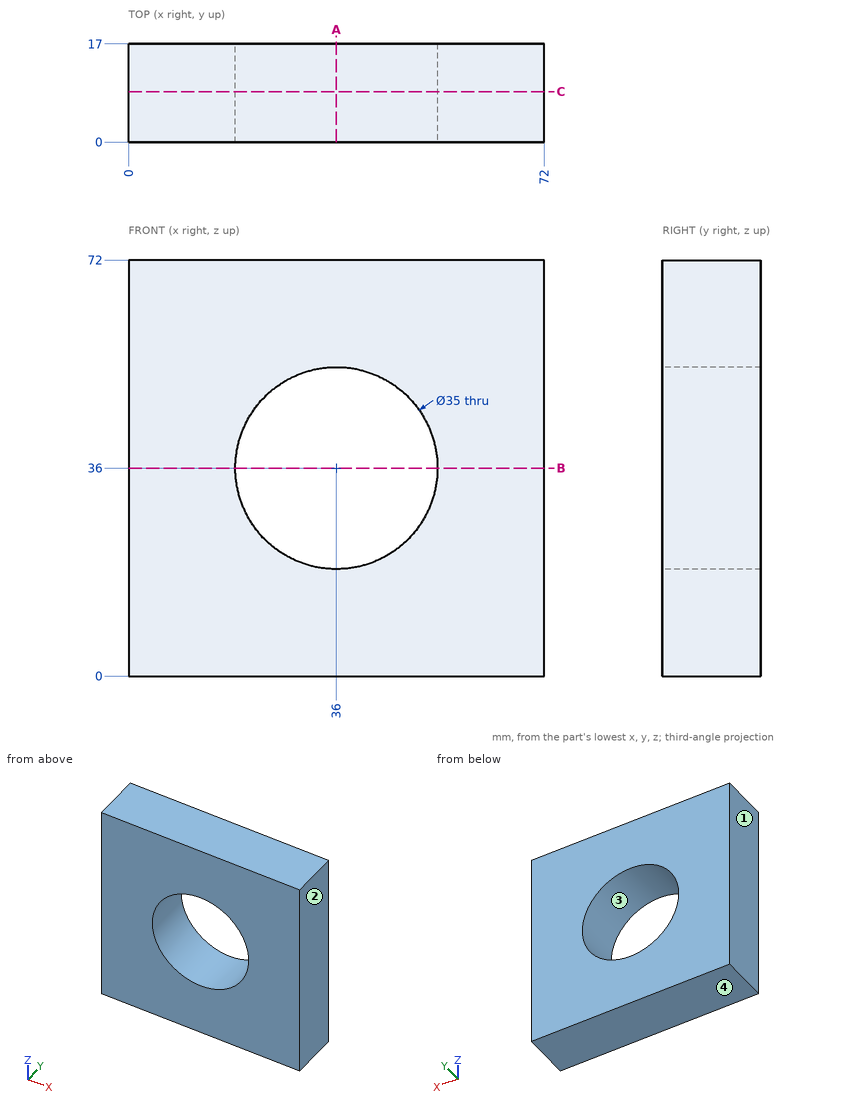
Geometry: see drawing. Coordinates: mm, zero at the bounding-box minimum. Give positions to 0.01 mm unless a question says otherwise; leave off trailing zeros. Loops run counter-clockwise (first coordinate to the right, second up) from the corner with the lowest first, then second, coordinate; pieces in that order, holes last. Notation, with made-up numbers: (31.25, 8.25) -> (85.25, 8.25) arc R34 ccw to (85.25, 46.25) -> close; hole circle Ø6 at (27, 64). An arc over 180 degrees is marked (long way). Put each result on its own line as item: value.
1. Pin query (flat end, axial travel): P1, Ø5, axis at x = 46.5, y = 5.5, coming from the -Z side. Return the tip coordinate at first contact, or that it passes through.
Taken from the geometry:
P1: stops at z = 0
2. Pull-direction query (X, two-part tool) for the marked faces 1, 2, 3 and 4; classes: released by +X, released by -X, zero draft, split by the parting line, or undercut.
Taken from the geometry:
face 1: released by -X
face 2: released by +X
face 3: undercut
face 4: zero draft
3. Ray query, line 1 along Z through (x, y) = (36, 7.75); line 2 along X through (y, z) = (12.5, 28); line 3 along X through (y, z) = (7.5, 23.5). Return the intervals inside material, ascending. Write a range as [from, to].
Taken from the geometry:
line 1: z = [0, 18.5], [53.5, 72]
line 2: x = [0, 20.44], [51.56, 72]
line 3: x = [0, 23.75], [48.25, 72]
4. Cut plane B-B (z = 36). Return the cut outline in (x, y).
Taken from the geometry:
outline: (0, 0) -> (18.5, 0) -> (18.5, 17) -> (0, 17) -> close; (53.5, 0) -> (72, 0) -> (72, 17) -> (53.5, 17) -> close
5. Cut plane C-C (y = 8.75). Return the cut outline in (x, z).
Taken from the geometry:
outline: (0, 0) -> (72, 0) -> (72, 72) -> (0, 72) -> close; hole circle Ø35 at (36, 36)
6. Cut plane A-A (x = 36). Return the cut outline in (y, z).
Taken from the geometry:
outline: (0, 0) -> (17, 0) -> (17, 18.5) -> (0, 18.5) -> close; (0, 53.5) -> (17, 53.5) -> (17, 72) -> (0, 72) -> close
